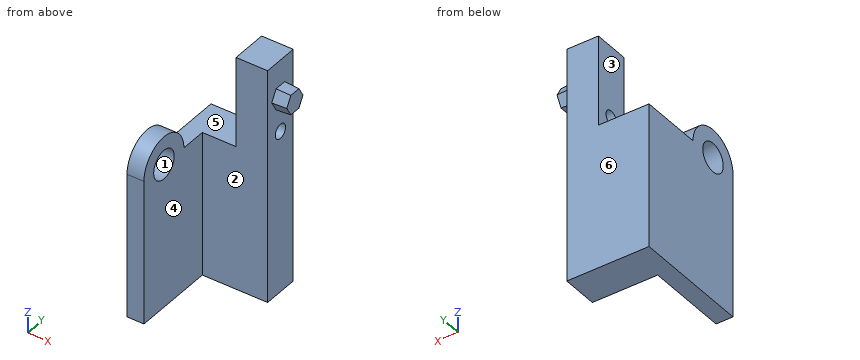
```python
from build123d import *

# Parameters (mm, degrees)
F0_W      = 12.7
F0_H      = 50.8
F1_DEPTH  = 11.0998
F3_DEPTH  = 5.08
F3_TAPER  = 3
F4_R      = 2.54
F5_DEPTH  = 16.1808001
F6_W      = 12.7
F6_H      = 19.05
F7_DEPTH  = 17.78
F8_W      = 5.9436
F8_H      = 19.05
F9_DEPTH  = 25.4
F10_W     = 5.9436
F10_H     = 12.7
F11_DEPTH = 6.35
F12_R     = 6.34999
F13_R     = 5.08
F14_DEPTH = 33.9608001
F16_DEPTH = 5.9436
F18_DEPTH = 31.75


# Not quite as in the source:
# - a fillet or chamfer is up to 0.001 mm smaller than in the source, because OpenCascade refuses the exact size


with BuildPart() as f1:
    # F0 (on Right) → F1 (new body)
    with BuildSketch(Plane.YZ):
        with Locations((6.35, 25.4)):
            Rectangle(F0_W, F0_H)
    extrude(amount=F1_DEPTH)

    # F2 (on face) → F3 (join)
    with BuildSketch(Plane.YZ.offset(11.0998)):
        Polygon((4.191, 34.3605023065), (8.509, 34.3605023065), (10.668, 38.1), (8.509, 41.8394976935), (4.191, 41.8394976935), (2.032, 38.1), align=None)
    extrude(amount=F3_DEPTH, taper=F3_TAPER)

    # F4 (on face) → F5 (cut, through all)
    with BuildSketch(Plane(origin=(0, 0, 0), x_dir=(0, -1, 0), z_dir=(-1, 0, 0))):
        with Locations((-6.35, 25.4)):
            Circle(F4_R)
    extrude(amount=-F5_DEPTH, mode=Mode.SUBTRACT)

    # F6 (on face) → F7 (join)
    with BuildSketch(Plane(origin=(0, 0, 0), x_dir=(0, -1, 0), z_dir=(-1, 0, 0))):
        with Locations((-6.35, 9.525)):
            Rectangle(F6_W, F6_H)
    extrude(amount=F7_DEPTH)

    # F8 (on face) → F9 (join)
    with BuildSketch(Plane.XZ):
        with Locations((-14.8082, 9.525)):
            Rectangle(F8_W, F8_H)
    extrude(amount=F9_DEPTH)

    # F10 (on face) → F11 (join)
    with BuildSketch(Plane.XY.offset(19.05)):
        with Locations((-14.8082, -19.05)):
            Rectangle(F10_W, F10_H)
    extrude(amount=F11_DEPTH)

    # F12 (radius 6.35 in the source; OpenCascade refuses exactly that, so slightly less here)
    f12_edges = [f1.edges().sort_by_distance(p)[0] for p in [
        (-14.8082, -12.7, 25.4),
        (-14.8082, -25.4, 25.4),
    ]]
    fillet(f12_edges, radius=F12_R)

    # F13 (on face) → F14 (cut, through all)
    with BuildSketch(Plane(origin=(-17.78, 0, 0), x_dir=(0, -1, 0), z_dir=(-1, 0, 0))):
        with Locations((19.05, 19.05)):
            Circle(F13_R)
    extrude(amount=-F14_DEPTH, mode=Mode.SUBTRACT)

    # F15 (on face) → F16 (join, through all)
    with BuildSketch(Plane(origin=(-17.78, 0, 0), x_dir=(0, -1, 0), z_dir=(-1, 0, 0))):
        with BuildLine():
            Line((28.956, 0), (28.956, 19.05))
            ThreePointArc((28.956, 19.05), (19.05, 28.956), (9.144, 19.05))
            Line((9.144, 19.05), (12.7, 19.05))
            ThreePointArc((12.7, 19.05), (19.05, 25.4), (25.4, 19.05))
            Line((25.4, 19.05), (25.4, 0))
            Line((25.4, 0), (28.956, 0))
        make_face()
    extrude(amount=-F16_DEPTH)

    # F17 (on face) → F18 (join)
    with BuildSketch(Plane(origin=(0, 0, 0), x_dir=(1, 0, 0), z_dir=(0, 0, -1))):
        Polygon((-17.78, -12.7), (11.0998, -12.7), (11.0998, 0), (-11.8364, 0), (-11.8364, 28.956), (-17.78, 28.956), align=None)
    extrude(amount=F18_DEPTH)


solid = f1.part
```
Check sheet for the modelled part. Datum: model origin and axes. Units: mm. Face numbers are marked on the shaded views. A direction names the side the tool comes from. Round coordinates to 2 decimals unless told otherwise and drop trailing zeros. Order: outer loops, then holes, each group sorted by start corner. A loop starts at its lowest first (then second) coordinate and runs counter-clockwise, first axis right, second up. Notation, with made-up numbers: M -27.5,6.25 L 29.5,6.25 A19 cw 29.5,27.25 Z; hole C 3.25,-9 d1. An arc over 180 degrees is marked long. Answer in a Markdown table with one row per item.
(1) Draft check along Y on the marked faces 1, 2 and 3. Enter one of: +Y half, -Y half, draft (parallel to the pull), parting line (faces both ways), or undercut.
Findings:
| item | result |
|---|---|
| face 1 | undercut |
| face 2 | -Y half |
| face 3 | draft |
(2) Section check B-B on z = 15.5. Record the boundary of the cut face in (x, y).
Findings:
| item | result |
|---|---|
| outline | M -17.78,-28.96 L -11.84,-28.96 L -11.84,-22.68 L -17.78,-22.68 Z; M -17.78,-15.42 L -11.84,-15.42 L -11.84,0 L 11.1,0 L 11.1,12.7 L -17.78,12.7 Z |
(3) Section check A-A on y = -16. Record the boundary of the cut face in (x, z), plus the area to 3 significant figures.
Findings:
| item | result |
|---|---|
| outline | M -17.78,-31.75 L -11.84,-31.75 L -11.84,14.99 L -17.78,14.99 Z; M -17.78,23.11 L -11.84,23.11 L -11.84,28.47 L -17.78,28.47 Z |
| area | 310 mm^2 |
(4) Set-up check for the marked faces 4, 5 and 6: record each of +Z, -Z, +X, -X, +Y, -Y from which the full face is reachable in a straight line by a thin tool's end or side.
Findings:
| item | result |
|---|---|
| face 4 | +Z, -Z, +X, -Y |
| face 5 | +Z, -X, +Y |
| face 6 | +Z, -Z, +X, -X, +Y |
(5) Section check D-D on z = 25.4. Record the boundary of the cut face in (x, y), plus the area to 3 significant figures.
Findings:
| item | result |
|---|---|
| outline | M -17.78,-26.65 L -11.84,-26.65 L -11.84,-11.45 L -17.78,-11.45 Z; M 0,0 L 11.1,0 L 11.1,3.81 L 0,3.81 Z; M 0,8.89 L 11.1,8.89 L 11.1,12.7 L 0,12.7 Z |
| area | 175 mm^2 |
(6) Gauge pin test, flat ends, axial feed: pin 1 (4 mm diameter, centred on x = -5.5, z = 13.5, fed in from -Y); pin 2 (5.5 mm diameter, centred on x = -11.5, y = 6, fed in from +Z); pin 3 (12 mm diameter, centred on x = -6.5, y = -19, fed in from +Z). Record the tip position at first contact, or that the pin passes through.
Findings:
| item | result |
|---|---|
| pin 1 | stops at y = 0 |
| pin 2 | stops at z = 19.05 |
| pin 3 | stops at z = 28.96 |
(7) Material ranges on line 1 along Z through (x, y) = (-14, -19); line 2 along Z through (x, y) = (6.25, 6.35); line 3 along X through (y, z) = (-3, -26.5), recorded low to high. Write a range as from..to.
Findings:
| item | result |
|---|---|
| line 1 | z = -31.75..13.97, 24.13..28.96 |
| line 2 | z = -31.75..22.86, 27.94..50.8 |
| line 3 | x = -17.78..-11.84 |
(8) Section check C-C on x = 8.5. Record the boundary of the cut face in (y, z), plus the area to 3 significant figures.
Findings:
| item | result |
|---|---|
| outline | M 0,-31.75 L 12.7,-31.75 L 12.7,50.8 L 0,50.8 Z; hole C 6.35,25.4 d5.08 |
| area | 1,030 mm^2 |
